Source: CAD feature listing. Evaluate the final solid. Frame: model axes, mm. Face numbers are marked on the shaded views. A direction names the side the tool comes from. Round coordinates to 2 decimals unless told otherwise and drop trailing zeros. Order: outer loops, then holes, each group sorted by start corner. A loop starts at its lowest first (then second) coordinate and runs counter-clockwise, first axis right, second up. Notation, with made-up numbers: M -28,42 L 10,42 A20 ccw 10,61 Z; hole C 82.5,35 d3. An arc over 180 degrees is marked long. Answer as CSV lines item,"result". Start each with the question number.
Item 1: Section query C-C on z = 92. Return the cut outline in (x, y).
Item 2: First-contact query: P1, Ø10, axis at x = 22.5, y = 27.5, coming from the +Z side; P2, Ø1.5, axis at x = -44, y = 9.5, coming from the -Z side. Flat tips, straight axial feed; report the tip coordinate or a pass-through.
Item 3: Section query D-D on y = 0. Return the cut outline in (x, z), plus the area to 3 significant figures.
Item 4: Section query B-B on y = -11. Return the cut outline in (x, z).
Item 5: Section query A-A on x = -28. Return the cut outline in (y, z), plus the area to 3 significant figures.
Item 6: Pull-direction query (Y, two-part tool) for the marked faces 1, 2 and 3; classes: +Y half, -Y half, draft (parallel to the pull), parting line (faces both ways), or undercut.
Item 7: Line query: line 1 (X direction, y = -2, z = 48); line 2 (Y direction, x = -8, z = 118.5). Output: solid intervals per line, ascending. Write a range as [from, to].
Item 8: Set-up query: the marked faces 4 and 5. Return all of +Z, -Z, +X, -X, +Y, -Y with unobstructed straight access to the full face (end or side cutting, diameter ignored); none if empty.
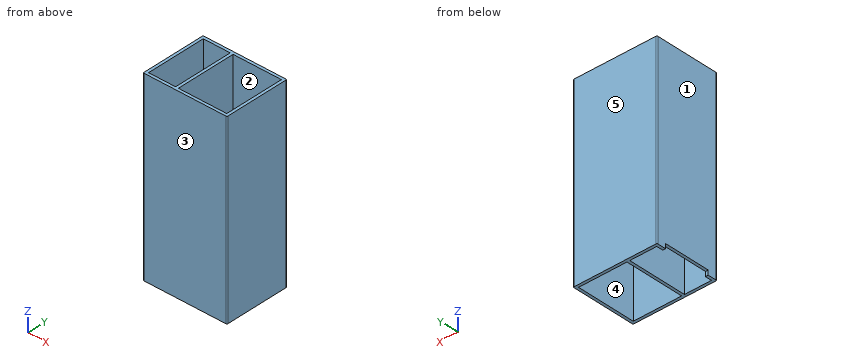
from build123d import *

# Parameters (mm, degrees)
ESBO_O1_W                = 90
ESBO_O1_H                = 70
ESBO_O1_W_2              = 29
ESBO_O1_H_2              = 64
ESBO_O1_W_3              = 52
RESSALTO_EXTRUS_O1_DEPTH = 200
FILETE1_R                = 1
ESBO_O4_R                = 4.75
ESBO_O4_R_2              = 2
CORTE_EXTRUS_O1_DEPTH    = 3
ESBO_O5_W                = 10.309676721
ESBO_O5_H                = 50
CORTE_EXTRUS_O2_DEPTH    = 5


with BuildPart() as part:
    # Esboço1 → Ressalto-extrusão1 (new body)
    with BuildSketch(Plane.XY):
        Rectangle(ESBO_O1_W, ESBO_O1_H)
        with Locations((-27.5, 0)):
            Rectangle(ESBO_O1_W_2, ESBO_O1_H_2, mode=Mode.SUBTRACT)
        with Locations((16, 0)):
            Rectangle(ESBO_O1_W_3, ESBO_O1_H_2, mode=Mode.SUBTRACT)
    extrude(amount=RESSALTO_EXTRUS_O1_DEPTH)

    # Filete1
    filete1_edges = [part.edges().sort_by_distance(p)[0] for p in [
        (45, -35, 100),
        (-45, -35, 100),
        (-45, 35, 100),
        (45, 35, 100),
    ]]
    fillet(filete1_edges, radius=FILETE1_R)

    # Esboço4 → Corte-extrusão1 (cut)
    with BuildSketch(Plane(origin=(-10, 0, 0), x_dir=(0, 0, -1), z_dir=(1, 0, 0))):
        with Locations(Location((-100, 0, 0), (0, 0, 90))):
            Circle(ESBO_O4_R)
        with Locations(Location((-92, 19.69381461, 0), (0, 0, 90))):
            Circle(ESBO_O4_R_2)
        with Locations(Location((-92, -16.897667481, 0), (0, 0, 90))):
            Circle(ESBO_O4_R_2)
    extrude(amount=-CORTE_EXTRUS_O1_DEPTH, mode=Mode.SUBTRACT)

    # Esboço5 → Corte-extrusão2 (cut)
    with BuildSketch(Plane(origin=(0, 0, 0), x_dir=(-1, 0, 0), z_dir=(0, 0, -1))):
        with Locations((43.55720026, 0)):
            Rectangle(ESBO_O5_W, ESBO_O5_H)
    extrude(amount=-CORTE_EXTRUS_O2_DEPTH, mode=Mode.SUBTRACT)


solid = part.part
Results:
1,outline,"M -45,-34 A1 ccw -44,-35 L 44,-35 A1 ccw 45,-34 L 45,34 A1 ccw 44,35 L -44,35 A1 ccw -45,34 Z; M -13,-14.9 L -10,-14.9 L -10,17.69 L -13,17.69 Z; hole M -42,-32 L -13,-32 L -13,-18.9 L -10,-18.9 L -10,-32 L 42,-32 L 42,32 L -10,32 L -10,21.69 L -13,21.69 L -13,32 L -42,32 Z"
2,P1,"z = 200"
2,P2,"z = 5"
3,outline,"M -45,5 L -42,5 L -42,200 L -45,200 Z; M -13,0 L -10,0 L -10,95.25 L -13,95.25 Z; M -13,104.75 L -10,104.75 L -10,200 L -13,200 Z; M 42,0 L 45,0 L 45,200 L 42,200 Z"
3,area,"1,760 mm^2"
4,outline,"M -45,5 L -42,5 L -42,200 L -45,200 Z; M -13,0 L -10,0 L -10,200 L -13,200 Z; M 42,0 L 45,0 L 45,200 L 42,200 Z"
5,outline,"M -35,0 L -32,0 L -32,200 L -35,200 Z; M 32,0 L 35,0 L 35,200 L 32,200 Z"
5,area,"1,200 mm^2"
6,face 1,"draft"
6,face 2,"undercut"
6,face 3,"-Y half"
7,line 1,"[-45, -42], [-13, -10], [42, 45]"
7,line 2,"[-35, -32], [32, 35]"
8,face 4,"+Z, -Z"
8,face 5,"+Z, -Z, +X, -X, +Y"
